```python
from build123d import *

# Parameters (mm, degrees)
SKETCH1_W           = 7
SKETCH1_H           = 7
BOSS_EXTRUDE1_DEPTH = 3
CUT_EXTRUDE1_DEPTH  = 7
CUT_EXTRUDE2_DEPTH  = 11
SKETCH4_R           = 1.8
CUT_EXTRUDE3_DEPTH  = 0.8
SKETCH5_W           = 0.961538462
SKETCH5_H           = 0.961538462
CUT_EXTRUDE4_DEPTH  = 0.4


with BuildPart() as part:
    # Sketch1 → Boss-Extrude1 (new body)
    with BuildSketch(Plane(origin=(0, 0, 0), x_dir=(1, 0, 0), z_dir=(0, 1, 0))):
        with Locations((3.5, 3.5)):
            Rectangle(SKETCH1_W, SKETCH1_H)
    extrude(amount=BOSS_EXTRUDE1_DEPTH)

    # Sketch2 → Cut-Extrude1 (cut)
    with BuildSketch(Plane.XY):
        Polygon((0, 0), (0.7, 3), (0, 3), align=None)
        Polygon((7, 0), (6.3, 3), (7, 3), align=None)
    extrude(amount=-CUT_EXTRUDE1_DEPTH, mode=Mode.SUBTRACT)

    # Sketch3 → Cut-Extrude2 (cut)
    with BuildSketch(Plane(origin=(0, 0, 0), x_dir=(0, 0, -1), z_dir=(1, 0, 0))):
        Polygon((0, 0), (0.7, 3), (0, 3), align=None)
        Polygon((7, 3), (6.3, 3), (7, 0), align=None)
    extrude(amount=CUT_EXTRUDE2_DEPTH, mode=Mode.SUBTRACT)

    # Sketch4 → Cut-Extrude3 (cut)
    with BuildSketch(Plane.XZ):
        with Locations(Location((3.5, -3.5, 0), (0, 0, 270))):
            Circle(SKETCH4_R)
    extrude(amount=-CUT_EXTRUDE3_DEPTH, mode=Mode.SUBTRACT)

    # Sketch5 → Cut-Extrude4 (cut)
    with BuildSketch(Plane(origin=(0, 3, 0), x_dir=(1, 0, 0), z_dir=(0, 1, 0))):
        with Locations((3.542267308, 3.542216335)):
            Rectangle(SKETCH5_W, SKETCH5_H)
    extrude(amount=-CUT_EXTRUDE4_DEPTH, mode=Mode.SUBTRACT)


solid = part.part
```
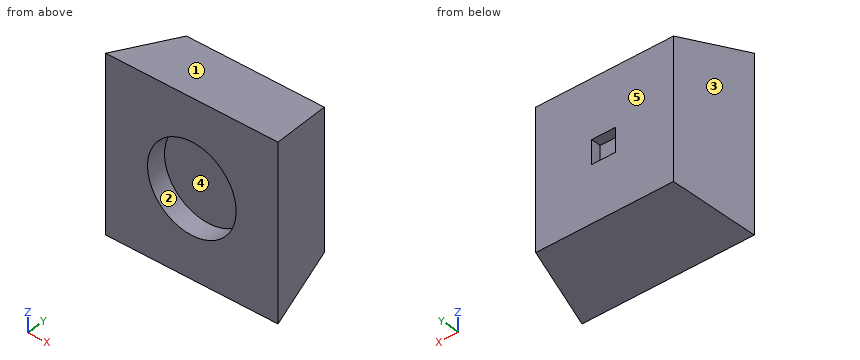
Part model, mm, in its own coordinate system. Face numbers are marked on the shaded views. A direction names the side the tool comes from. Give positions to 0.01 mm unless a question says otherwise; leave off trailing zeros. Order: outer loops, then holes, each group sorted by start corner. A loop starts at its lowest first (then second) coordinate and runs counter-clockwise, first axis right, second up. Notation, with made-up numbers: M 63.5,49 L 80.5,49 A28 ccw 80.5,74 Z; hole C 9,16.25 d3. An arc over 180 degrees is marked long. Use a Markdown table: item, result. Add a question column.
(1) Saw through at D-D, the plane z = -2.5. Give the cut face in (x, y).
(2) 3-axis set-ups, long thin cutter, end or side, ignore diameter. For the marked faces 4 and 5: which of +Z, -Z, +X, -X, +Y, -Y reach the whole face in a straight line?
(3) Mould opens along X. For the marked faces 1, 2 and 3 say: +X half, -X half, draft (parallel to the pull), parting line (faces both ways), or undercut.
(4) Saw through at C-C, the plane y = 0.5. Give the cut face in (x, z).
(5) Probe line 1 along Y through (x, z) = (3.75, -3); line 2 along X through (y, z) = (0.4, -3.5); line 3 along X through (y, z) = (0.9, -4.5). List the from-to ranges inside material, lowest first. Write a range as [from, to].
(6) Saw through at B-B, the plane x = 3.5. Give the cut face in (y, z), and give its area (3 significant figures).
(7) Saw through at A-A, the plane z = -3.5. Give the cut face in (x, y), and give its area (3 significant figures).
(8) Drop flat-ended pins along their axis: P1, Ø2, axis at x = 3.5, z = -3.5, coming from the -Y side; P2, Ø0.8, axis at x = 3.5, z = -3.5, coming from the +Y side; P3, Ø1, axis at y = 1.5, z = -3, coming from the +X side. Give the stop position or say it passes through.
Answer key:
| question | item | result |
|---|---|---|
| 1 | outline | M 0,0 L 2,0 L 2,0.8 L 5,0.8 L 5,0 L 7,0 L 6.3,3 L 0.7,3 Z |
| 2 | face 4 | -Y |
| 2 | face 5 | +Z, -Z, +X, -X, +Y |
| 3 | face 1 | draft |
| 3 | face 2 | undercut |
| 3 | face 3 | -X half |
| 4 | outline | M 0.12,-6.88 L 6.88,-6.88 L 6.88,-0.12 L 0.12,-0.12 Z; hole C 3.5,-3.5 d3.6 |
| 5 | line 1 | [0.8, 3] |
| 5 | line 2 | [0.09, 1.7], [5.3, 6.91] |
| 5 | line 3 | [0.21, 6.79] |
| 6 | outline | M 0,-7 L 3,-6.3 L 3,-4.02 L 2.6,-4.02 L 2.6,-3.06 L 3,-3.06 L 3,-0.7 L 0,0 L 0,-1.7 L 0.8,-1.7 L 0.8,-5.3 L 0,-5.3 Z |
| 6 | area | 15.6 mm^2 |
| 7 | outline | M 0,0 L 1.7,0 L 1.7,0.8 L 5.3,0.8 L 5.3,0 L 7,0 L 6.3,3 L 4.02,3 L 4.02,2.6 L 3.06,2.6 L 3.06,3 L 0.7,3 Z |
| 7 | area | 15.6 mm^2 |
| 8 | P1 | y = 0.8 |
| 8 | P2 | y = 2.6 |
| 8 | P3 | x = 6.77 |
